Autodesk Fusion 360 part; units mm, degrees
sketch "Sketch1" plane through (0, 0, 0) normal (0, 0, 1) x (1, 0, 0)
  line L0 (0, 2.7263) -> (0, 35)
  line L1 (2.3029, 1.4592) -> (9.9175, 6.2842)
  arc A0 (9.9175, 6.2842) -> (11.71, 18.2478) centre (5.6356, 13.0418) ccw
  line L2 (11.71, 18.2478) -> (3.2204, 28.1536)
  arc A1 (3.9309, 34.0102) -> (3.2204, 28.1536) centre (6.2576, 30.7565) ccw
  line L3 (3.9309, 34.0102) -> (7.0243, 35.9704)
  line L4 (-1.2, 35) -> (0, 35)
  line L5 (7.0243, 35.9704) -> (7.6666, 34.9567)
  arc A2 (0, 2.7263) -> (2.3029, 1.4592) centre (1.5, 2.7263) ccw
  line L6 (4.6041, 33.0162) -> (7.6666, 34.9567)
  arc A3 (4.6041, 33.0162) -> (4.1316, 28.9345) centre (6.2576, 30.7565) ccw
  line L7 (12.6211, 19.0286) -> (4.1316, 28.9345)
  arc A4 (10.5598, 5.2706) -> (12.6211, 19.0286) centre (5.6356, 13.0418) ccw
  line L8 (2.9452, 0.4456) -> (10.5598, 5.2706)
  arc A5 (-1.2, 2.7263) -> (2.9452, 0.4456) centre (1.5, 2.7263) ccw
  line L9 (-1.2, 2.7263) -> (-1.2, 35)
  dimension "d1" = 35
  dimension "d2" = 8
  dimension "d3" = 4
  dimension "d4" = -1.2
  dimension "d7" = 1.5
extrude "Extrude1" add sketch "Sketch1" along normal blind 32
Verification items for the finished model (mm, model axes). A direction names the side the tool comes from. Give positions to 0.01 mm unless a question says otherwise; leave off trailing zeros. Loops run counter-clockwise (first coordinate to the right, second up) from the corner with the lowest first, then second, coordinate; pieces in that order, holes last. Notation, with made-up numbers: M 72.25,-25.75 L 122.25,-25.75 A26 ccw 122.25,-10.75 Z; hole C -21.5,57.25 d7. An arc over 180 degrees is marked long. One line per question, with ' | ' between items.
Item 1: Draft check along Y on faces 1 (the face through (-0.3, 15.4, 0)), 2 (the face through (13.56, 11.95, 15.78)), 3 (the face through (6.699, 2.824, 15.776)), 4 (the face through (2.28, 31.19, 15.78)). Enter one of: +Y half, -Y half, draft (parallel to the pull), parting line (faces both ways), or undercut.
Completed:
face 1: draft | face 2: undercut | face 3: -Y half | face 4: undercut
Item 2: Section check D-D, the plane x = 0.75. Record the cut outline in (y, z).
Completed:
outline: M 0.13,0 L 1.43,0 L 1.43,32 L 0.13,32 Z
Item 3: Section check A-A, the plane y = 7. Record the cut outline in (x, z).
Completed:
outline: M -1.2,0 L 0,0 L 0,32 L -1.2,32 Z; M 10.88,0 L 12.57,0 L 12.57,32 L 10.88,32 Z
Item 4: Section check B-B, the plane z = 30. Record the cut outline in (x, y).
Completed:
outline: M -1.2,2.73 A2.7 ccw 2.95,0.45 L 10.56,5.27 A9.2 ccw 12.62,19.03 L 4.13,28.93 A2.8 cw 4.6,33.02 L 7.67,34.96 L 7.02,35.97 L 3.93,34.01 A4 ccw 3.22,28.15 L 11.71,18.25 A8 cw 9.92,6.28 L 2.3,1.46 A1.5 cw 0,2.73 L 0,35 L -1.2,35 Z
Item 5: Thickness scan on line 1 (Y direction, x = 5.75, z = 20); line 2 (Y direction, x = 7, z = 24) (1 decimal); line 3 (X direction, y = 11, z = 29). Record the ranges inside material, lowest first. Write a range as [from, to].
Completed:
line 1: y = [2.22, 3.64], [25.2, 27.05], [33.74, 35.16] | line 2: y = [3, 4.4], [23.7, 25.6], [34.5, 36] | line 3: x = [-1.2, 0], [13.37, 14.61]
Item 6: Section check C-C, the plane x = 9.5. Record the cut outline in (y, z), plus the area to 3 significant figures.
Completed:
outline: M 4.6,0 L 6.02,0 L 6.02,32 L 4.6,32 Z; M 20.83,0 L 22.67,0 L 22.67,32 L 20.83,32 Z | area: 104 mm^2
Item 7: Tool access check on faces 5 (the face through (6.06, 3.84, 15.78)), 6 (the face through (5.46, 34.98, 15.78)), 7 (the face through (8.44, 23.91, 15.78)), 8 (the face through (-1, 35, 16)). Record the directions out of +Z, -Z, +X, -X, +Y, -Y that give a thin tool (end or side, any length) a straight path to the whole face; none if there is none.
Completed:
face 5: +Z, -Z | face 6: +Z, -Z, +Y | face 7: +Z, -Z, +X | face 8: +Z, -Z, -X, +Y
Item 8: Depth check by flat-ended pin: P1, Ø4, axis at x = 11.5, z = 16, coming from the -Y side; P2, Ø4, axis at x = 9.5, y = 4, coming from the -Z side; P3, Ø2, axis at y = 23, z = 9.5, coming from the +X side; P4, Ø1.5, axis at x = 6, z = 24, coming from the +Y side. Enter the tip coordinate at first touch or a pass-through.
Completed:
P1: stops at y = 4.6 | P2: stops at z = 0 | P3: stops at x = 10.07 | P4: stops at y = 35.8
